```python
from build123d import *

# Parameters (mm, degrees)
SKETCH1_R                   = 6.35
BOSS_EXTRUDE1_DEPTH         = 91.0844
F_1_4_20_TAPPED_HOLE1_D     = 5.1054
F_1_4_20_TAPPED_HOLE1_DEPTH = 25.4
F_1_4_20_TAPPED_HOLE1_TIP   = 1.533816902
F_1_4_20_TAPPED_HOLE2_D     = 5.1054
F_1_4_20_TAPPED_HOLE2_DEPTH = 25.4
F_1_4_20_TAPPED_HOLE2_TIP   = 1.533816902


with BuildPart() as part:
    # Sketch1 → Boss-Extrude1 (new body)
    with BuildSketch(Plane(origin=(0, 0, 0), x_dir=(1, 0, 0), z_dir=(0, 1, 0))):
        with Locations(Location((0, 0, 0), (0, 0, 270))):
            Circle(SKETCH1_R)
    extrude(amount=BOSS_EXTRUDE1_DEPTH)

    # 1/4-20 Tapped Hole1
    with Locations(Plane(origin=(0, 91.0844, 0), x_dir=(1, 0, 0), z_dir=(0, 1, 0))):
        with Locations((0, 0)):
            Hole(F_1_4_20_TAPPED_HOLE1_D / 2, depth=F_1_4_20_TAPPED_HOLE1_DEPTH)
            with Locations((0, 0, -(F_1_4_20_TAPPED_HOLE1_DEPTH + F_1_4_20_TAPPED_HOLE1_TIP / 2))):  # 118° drill point
                Cone(0, F_1_4_20_TAPPED_HOLE1_D / 2, F_1_4_20_TAPPED_HOLE1_TIP, mode=Mode.SUBTRACT)

    # 1/4-20 Tapped Hole2
    with Locations(Plane(origin=(0, 0, 0), x_dir=(-1, 0, 0), z_dir=(0, -1, 0))):
        with Locations((0, 0)):
            Hole(F_1_4_20_TAPPED_HOLE2_D / 2, depth=F_1_4_20_TAPPED_HOLE2_DEPTH)
            with Locations((0, 0, -(F_1_4_20_TAPPED_HOLE2_DEPTH + F_1_4_20_TAPPED_HOLE2_TIP / 2))):  # 118° drill point
                Cone(0, F_1_4_20_TAPPED_HOLE2_D / 2, F_1_4_20_TAPPED_HOLE2_TIP, mode=Mode.SUBTRACT)


solid = part.part
```
Part model, mm, in its own coordinate system. A direction names the side the tool comes from. Coordinates: 2 decimals unless noted, no trailing zeros. Loops run counter-clockwise (first coordinate to the right, second up) from the corner with the lowest first, then second, coordinate; pieces in that order, holes last. Notation, with made-up numbers: (38, 42.5) - (90, 42.5) arc R15 cw to (90, 67.5) - close; hole circle Ø11 at (12, -33.75). An arc over 180 degrees is marked (long way). Write item = value, one per line. Start each with the question number.
Item 1: Cut at B-B, the plane x = -3.5. Give the cut face in (y, z), and give its area (3 significant figures).
Item 2: Cut at D-D, the plane x = 4.75. Give the cut face in (y, z).
Item 3: Mould opens along Z. For faces 1 (the cylindrical face through (-3.86, 44.9, -5.04)), 2 (the flat face through (0, 0, 3)), 3 (the cylindrical face through (2.435, 12.878, -0.767)) say: released by +Z, released by -Z, zero draft, split by the parting line, or undercut.
Item 4: Cut at A-A, the plane y = 13.5. Give the cut face in (x, z), and give its area (3 significant figures).
Item 5: Flat gauge pins, fed straight in: pin 1 Ø5 at (x, z) = (2.5, -2.5) entering from -Y; pin 2 Ø1 at (y, z) = (21.5, 2.5) entering from -X. Where does each tip first touch, or does it go through?
Item 6: Wall check: L1, parallel to X at y = 20, z = -1.75; L2, parallel to X at y = 72, z = 0.25; L3, parallel to Z at x = -1.5, y = 45. Give the ranges that are in metal, low to high. Write a range as from..to.
Item 7: 3-axis set-ups, long thin cutter, end or side, ignore diameter. For faces 4 (the cylindrical face through (-2.435, 78.207, -0.767)), 5 (the flat face through (0, 91.084, 3)): which of +Z, -Z, +X, -X, +Y, -Y reach the whole face in a straight line?
Item 8: Cut at C-C, the plane y = 51. Give the cut face in (x, z), and give its area (3 significant figures).
The answers:
q1.outline = (0, -5.3) - (91.08, -5.3) - (91.08, 5.3) - (0, 5.3) - close
q1.area = 965 mm2
q2.outline = (0, -4.21) - (91.08, -4.21) - (91.08, 4.21) - (0, 4.21) - close
q3.face_1 = split by the parting line
q3.face_2 = zero draft
q3.face_3 = undercut
q4.outline = circle Ø12.7 at (0, 0); hole circle Ø5.11 at (0, 0)
q4.area = 106 mm2
q5.pin_1 = 0
q5.pin_2 = -6.03
q6.L1 = -6.1..-1.86, 1.86..6.1
q6.L2 = -6.35..-2.54, 2.54..6.35
q6.L3 = -6.17..6.17
q7.face_4 = +Y
q7.face_5 = +Z, -Z, +X, -X, +Y
q8.outline = circle Ø12.7 at (0, 0)
q8.area = 127 mm2
